Input: part model. Units: mm. Frame: model coordinates. Face numbers are marked on the shaded views. A direction names the side the tool comes from. Give positions to 0.01 mm unless a question says otherwise; leave off trailing zeros. Loops run counter-clockwise (first coordinate to the right, second up) from the corner with the lowest first, then second, coordinate; pieces in that order, holes last. Notation, with made-up numbers: M 2,-27.5 L 50,-27.5 A15 ccw 50,-11.5 Z; hole C -12.75,10.25 d3. An arc over 180 degrees is marked long. Use a Markdown table: item, result. Add a question column.
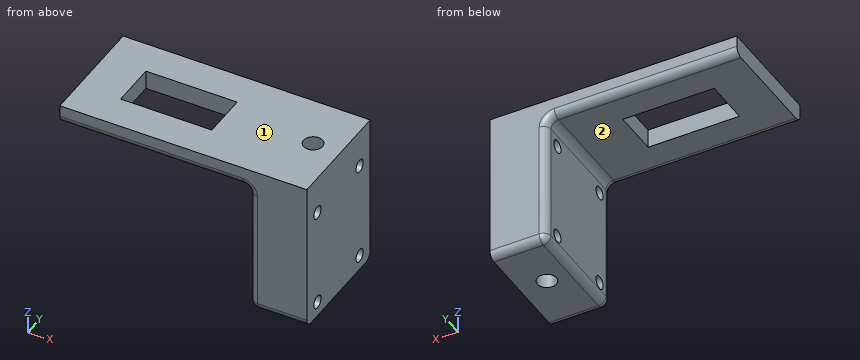
Autodesk Inventor part; units mm, degrees
ref_plane "YZ Plane" through (0, 0, 0) normal (1, 0, 0) x (0, 1, 0)
ref_plane "XZ Plane" through (0, 0, 0) normal (0, 1, 0) x (-1, 0, 0)
ref_plane "XY Plane" through (0, 0, 0) normal (0, 0, 1) x (1, 0, 0)
sketch "Skizze1" plane through (0, 0, 0) normal (0, 1, 0) x (-1, 0, 0)
  line L0 (65, 5.2632) -> (0, 5.2632)
  line L1 (0, 5.2632) -> (0, -34.7368)
  line L2 (0, -34.7368) -> (15, -34.7368)
  line L3 (15, -34.7368) -> (15, 0.2632)
  line L4 (15, 0.2632) -> (65, 0.2632)
  line L5 (65, 0.2632) -> (65, 5.2632)
  point P0 (0, 0)
  dimension "d0" = 5
  dimension "d1" = 15
  dimension "d2" = 40
  dimension "d5" = 65
extrude "Extrusion1" add sketch "Skizze1" along normal blind 30
sketch "Skizze2" plane through (-65, 0, 5.2632) normal (0, 0, 1) x (1, 0, 0)
  line L0 (11, 9) -> (35, 9)
  line L1 (35, 9) -> (35, 21)
  line L2 (35, 21) -> (11, 21)
  line L3 (11, 21) -> (11, 9)
  line L4 (65, 0) -> (65, 30)
  line L5 (0, 30) -> (65, 30)
  dimension "d6" = 30
  dimension "d7" = 24
  dimension "d8" = 12
  dimension "d9" = 9
extrude "Extrusion2" cut sketch "Skizze2" against normal blind 5
sketch "Skizze3" plane through (0, 0, 5.2632) normal (1, 0, 0) x (0, 0, -1)
  circle A0 centre (10, 5) radius 1.7
  circle A1 centre (36, 5) radius 1.7
  circle A2 centre (10, 25) radius 1.7
  circle A3 centre (36, 25) radius 1.7
  line L0 (0, 0) -> (0, 30)
  line L1 (0, 30) -> (40, 30)
  line L2 (40, 0) -> (40, 30)
  point P0 (5.2632, 0)
  dimension "d12" = 3.4
  dimension "d13" = 3.4
  dimension "d14" = 3.4
  dimension "d15" = 3.4
  dimension "d16" = 10
  dimension "d17" = 20
  dimension "d18" = 5
  dimension "d19" = 10
  dimension "d20" = 4
  dimension "d21" = 20
  dimension "d22" = 4
  dimension "d23" = 5
extrude "Extrusion3" cut sketch "Skizze3" against normal blind 20
sketch "Skizze4" plane through (0, 0, 5.2632) normal (1, 0, 0) x (0, 0, -1)
  point P0 (5.2632, 0)
sketch "Skizze5" plane through (0, 0, -34.7368) normal (0, 0, -1) x (-1, 0, 0)
  arc A0 (0.0007, -11.0976) -> (-0.0008, 42.9427) centre (7.2057, 15.9227) ccw
  circle A1 centre (7.2057, 15.9227) radius 2.5
  point P0 (0, 0)
  dimension "d26" = 5
extrude "Extrusion4" cut sketch "Skizze5" against normal through all
fillet "Rundung1" radius 2 8 edges at (-15, 30, -17.2368) (-15, 0, -17.2368) (-15, 15, -34.7368) (-40, 30, 0.2632) (-15, 15, 0.2632) (-40, 0, 0.2632) (-7.5, 30, -34.7368) (-7.5, 0, -34.7368)
properties part number "L-Halterung Servo"
1) Ray query, line 1 (X direction, y = 24.75, z = -21.5); line 2 (X direction, y = 15, z = -5); line 3 (X direction, y = 14, z = -6). Return the intervals inside material, ascending. Write a range as [from, to].
2) Section query A-A, the plane y = 5. Return the cut outline in (x, z), and give its area (3 significant figures).
3) Reachability of the marked faces 1 and 2 from +Z, -Z, +X, -X, +Y, -Y: full face, straight path, thin tool, end or side. Return the list, or none.
4) Section query B-B, the plane y = 10.5. Return the cut outline in (x, z).
5) Contact query for flat-ended pins moving along their axis: P1, Ø3, axis at y = 24, z = -30.5, coming from the +X side; P2, Ø10, axis at x = -51.5, z = -4.5, coming from the -Y side; P3, Ø4, axis at y = 5, z = -30.74, coming from the -X side. Output: stop coordinate, or through.
6) Section query D-D, the plane z = -18. Return the cut outline in (x, y).
7) Section query C-C, the plane x = -50. Return the cut outline in (y, z), and give its area (3 significant figures).
Entries:
| question | item | result |
|---|---|---|
| 1 | line 1 | x = [-15, 0] |
| 1 | line 2 | x = [-15, -9.53], [-4.88, 0] |
| 1 | line 3 | x = [-15, -8.8], [-5.61, 0] |
| 2 | outline | M -65,0.26 L -17,0.26 A2 cw -15,-1.74 L -15,-3.04 L 0,-3.04 L 0,5.26 L -65,5.26 Z; M -15,-32.74 A2 ccw -13,-34.74 L 0,-34.74 L 0,-32.44 L -15,-32.44 Z; M -15,-29.04 L 0,-29.04 L 0,-6.44 L -15,-6.44 Z |
| 2 | area | 748 mm² |
| 3 | face 1 | +Z, +X, -X, +Y, -Y |
| 3 | face 2 | -Z, -X, +Y, -Y |
| 4 | outline | M -65,0.26 L -54,0.26 L -54,5.26 L -65,5.26 Z; M -30,0.26 L -17,0.26 A2 cw -15,-1.74 L -15,-32.74 A2 ccw -13,-34.74 L 0,-34.74 L 0,5.26 L -30,5.26 Z |
| 5 | P1 | stops at x = 0 |
| 5 | P2 | stops at y = 1.06 |
| 5 | P3 | stops at x = -15 |
| 6 | outline | M -15,2 A2 ccw -13,0 L 0,0 L 0,30 L -13,30 A2 ccw -15,28 Z; hole C -7.21,15.92 d5 |
| 7 | outline | M 0,2.26 A2 ccw 2,0.26 L 9,0.26 L 9,5.26 L 0,5.26 Z; M 21,0.26 L 28,0.26 A2 ccw 30,2.26 L 30,5.26 L 21,5.26 Z |
| 7 | area | 88.3 mm² |
